Read the model definition and answer for the solid it produces. Units are mm, in the model's axes. A direction names the side the tool comes from. Coordinates: 2 decimals unless noted, no trailing zeros. Loops run counter-clockwise (first coordinate to the right, second up) from the corner with the lowest first, then second, coordinate; pieces in that order, holes last. Notation, with made-up numbers: (27.5, -2) - (42.5, -2) arc R13 ccw to (42.5, 8) - close; hole circle Ø3 at (-40, -7). An arc over 180 degrees is marked (long way). Use one line per item in the form item = value. Start each with the question number.
1) Which of the six approach directions +Z, -Z, +X, -X, +Y, -Y give full straight-line access (tool end or side, diameter ignored) to faces 5 (the face through (-16, -9, 5)), 6 (the face through (5.777, 0, -8)), 7 (the face through (0, -16, 12))?
2) The mould has two halves that part along X. Classify faces 1 (the face through (0, 0, 25)), 2 (the face through (-23, 15, 23)), 3 (the face through (-17.5, -9.07, 2.46)), 4 (the face through (-23, 2, 27)): released by +X, released by -X, zero draft, split by the parting line, or undercut.
3) A cutting plane is placed at D-D (z = 26). Give the vertices of the cut face in (x, y).
4) Consider line 1 (Y direction, x = -16, z = 2.3); line 2 (Y direction, x = 8, z = -11); line 3 (X direction, y = -8, z = 1.5). Determine where each line is inside the solid, lowest interval first.
5) Each of these flat-tipped pins is pushed along its axis until it touches: P1, Ø1.5, axis at x = -16.5, y = -8.5, coming from the -Z side; P2, Ø3.5, axis at x = -16.5, y = 9.5, coming from the -Z side; P3, Ø4, axis at x = 8, y = 0, coming from the -Z side; P4, Ø5, axis at x = -16, y = 9, coming from the +Z side. Where does it stop, or does it pass through?
6) A cutting plane is placed at C-C (x = -47.5). Give the vertices of the cut face in (y, z).
7) A cutting plane is placed at B-B (z = -4). Give the vertices of the cut face in (x, y), and give its area (3 significant figures).
8) A cutting plane is placed at A-A (x = 17). Give the vertices of the cut face in (y, z).
Autodesk Inventor part; units mm, degrees
ref_plane "YZ Plane" through (0, 0, 0) normal (1, 0, 0) x (0, 1, 0)
ref_plane "XZ Plane" through (0, 0, 0) normal (0, 1, 0) x (-1, 0, 0)
ref_plane "XY Plane" through (0, 0, 0) normal (0, 0, 1) x (1, 0, 0)
sketch "Sketch1" plane through (0, 0, 0) normal (0, 0, 1) x (1, 0, 0)
  line L0 (23, -16) -> (-23, -16)
  line L1 (-23, -16) -> (-23, 16)
  line L2 (-23, 16) -> (23, 16)
  line L3 (23, 16) -> (23, -16)
  line L4 (23, -16) -> (-23, 16) construction
  line L5 (-23, -16) -> (23, 16) construction
  line L6 (0, 0) -> (32.2248, 0) construction
  line L7 (0, 0) -> (0, 21.3704) construction
  circle A0 centre (8, 0) radius 3
  circle A1 centre (17, 9) radius 1.5
  circle A2 centre (-16, 9) radius 1.5
  line L8 (17, 9) -> (-16, 9) construction
  circle A3 centre (17, -9) radius 1.5
  circle A4 centre (-16, -9) radius 1.5
  line L9 (5.7769, -2.0144) -> (5.7769, 2.0144)
  dimension "d0" = 46
  dimension "d1" = 32
  dimension "d2" = 6
  dimension "d3" = 15
  dimension "d7" = 3
  dimension "d9" = 3
  dimension "d14" = 33
  dimension "d15" = 9
  dimension "d16" = 9
extrude "Extrusion1" add sketch "Sketch1" against normal blind 14 contours A0 L9 picked at (7.5179, 0)
extrude "Extrusion2" add sketch "Sketch1" against normal blind 2.5 contours A0 L9 | L9 A0
extrude "Extrusion3" add sketch "Sketch1" along normal blind 25 contours L0 L1 L2 L3 | A0 L9 | L9 A0 | A1 | A2 | A3 | A4
extrude "Extrusion4" cut sketch "Sketch1" along normal blind 5 contours A1 | A2 | A3 | A4
sketch "Sketch2" plane through (-23, -16, 0) normal (-1, 0, 0) x (0, 0, 1)
  circle A0 centre (16.25, 18.25) radius 13.75
  line L0 (0, 32) -> (25, 32)
  line L1 (0, 0) -> (0, 32)
  point P0 (0, 16)
  dimension "d23" = 27.5
  dimension "d24" = 16.25
extrude "Extrusion5" add sketch "Sketch2" along normal blind 45
sketch "Sketch3" plane through (0, 0, -14) normal (0, 0, -1) x (-1, 0, 0)
  arc A0 (-5.7769, 2.0144) -> (-5.7769, -2.0144) centre (-8, 0) ccw
  circle A1 centre (-8, 0) radius 1.5
  point P0 (0, 0)
  dimension "d29" = 3
extrude "Extrusion7" cut sketch "Sketch3" against normal blind 5
properties part number "motor"
Found:
q1.face_5 = -Z
q1.face_6 = -Z, -X, +Y, -Y
q1.face_7 = +Z, -Z, +X, -X, -Y
q2.face_1 = zero draft
q2.face_2 = released by -X
q2.face_3 = undercut
q2.face_4 = released by +X
q3.outline = (-68, -7.45) - (-23, -7.45) - (-23, 11.95) - (-68, 11.95) - close
q4.line_1 = -16 to -10.5, -7.5 to 7.5, 10.5 to 16
q4.line_2 = -3 to -1.5, 1.5 to 3
q4.line_3 = -23 to -17.12, -14.88 to 15.88, 18.12 to 23
q5.P1 = 5
q5.P2 = 0
q5.P3 = -14
q5.P4 = 25
q6.outline = circle Ø27.5 at (2.25, 16.25)
q7.outline = (5.78, -2.01) arc R3 ccw (long way) to (5.78, 2.01) - close
q7.area = 26.1 mm^2
q8.outline = (-16, 0) - (-10.5, 0) - (-10.5, 5) - (-7.5, 5) - (-7.5, 0) - (7.5, 0) - (7.5, 5) - (10.5, 5) - (10.5, 0) - (16, 0) - (16, 25) - (-16, 25) - close
